Job drawing, mm, ordinate dimensions from the low corner. One solid piece. Give positions to 0.01 mm unless a question says otherwise; leave off trailing zeros. Loops run counter-clockwise (first coordinate to the right, second up) from the corner with the lowest first, then second, coordinate; pieces in that order, holes last. Notation, with made-up numbers: M 9,41.5 L 56,41.5 A24 cw 56,66.5 Z; hole C -37,-31 d7. An arc over 180 degrees is marked long. Answer in a Markdown table with one row per item.
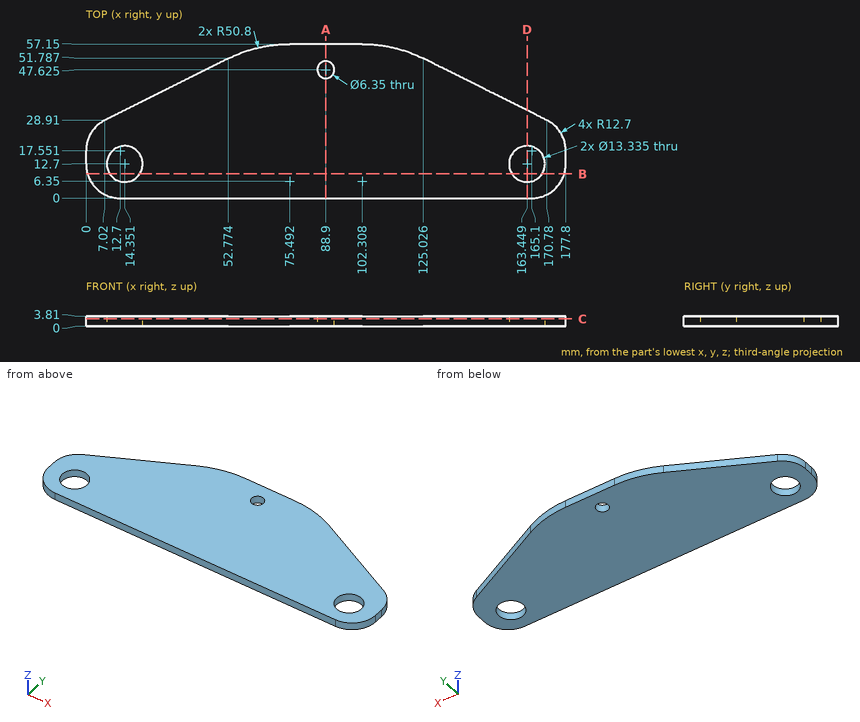
(1) Saw through at A-A (x = 88.9). Write the cut outline in (y, z).
Recorded:
| item | result |
|---|---|
| outline | M 0,0 L 44.45,0 L 44.45,3.81 L 0,3.81 Z; M 50.8,0 L 57.15,0 L 57.15,3.81 L 50.8,3.81 Z |
(2) Pin check, flat tips, straight feed: pin 1 Ø1.5 at (x, y) = (134, 48.5) entering from +Z; pin 2 Ø1.5 at (x, z) = (138.5, 0.5) entering from +Y (1 decimal). Stop position of each tip, or through.
Recorded:
| item | result |
|---|---|
| pin 1 | passes through |
| pin 2 | stops at y = 45.4 |
(3) Saw through at B-B (y = 9). Write the cut outline in (x, z) (1 decimal).
Recorded:
| item | result |
|---|---|
| outline | M 0.6,0 L 8.8,0 L 8.8,3.8 L 0.6,3.8 Z; M 19.9,0 L 157.9,0 L 157.9,3.8 L 19.9,3.8 Z; M 169,0 L 177.2,0 L 177.2,3.8 L 169,3.8 Z |
(4) Drill centre lines: line 1 along X through (y, z) = (10, 0.7) (1 decimal); line 2 along X through (y, z) = (18.5, 1) (1 decimal); line 3 along Y through (x, z) = (161, 0.3). Where is each one in solid material? Low to high.
Recorded:
| item | result |
|---|---|
| line 1 | x = 0.3 to 8.3, 20.4 to 157.4, 169.5 to 177.5 |
| line 2 | x = 0 to 11.1, 17.6 to 160.2, 166.7 to 177.8 |
| line 3 | y = 0 to 6.5, 18.9 to 33.8 |
(5) Saw through at C-C (z = 2.8). Give the number of separate pieces and of enclosed holes in the cut face, plus the area to 3 significant figures.
Recorded:
| item | result |
|---|---|
| separate pieces | 1 |
| enclosed holes | 3 |
| area | 7,720 mm^2 |
(6) Saw through at D-D (x = 163.5). Write the cut outline in (y, z).
Recorded:
| item | result |
|---|---|
| outline | M 0,0 L 6.03,0 L 6.03,3.81 L 0,3.81 Z; M 19.37,0 L 32.55,0 L 32.55,3.81 L 19.37,3.81 Z |
